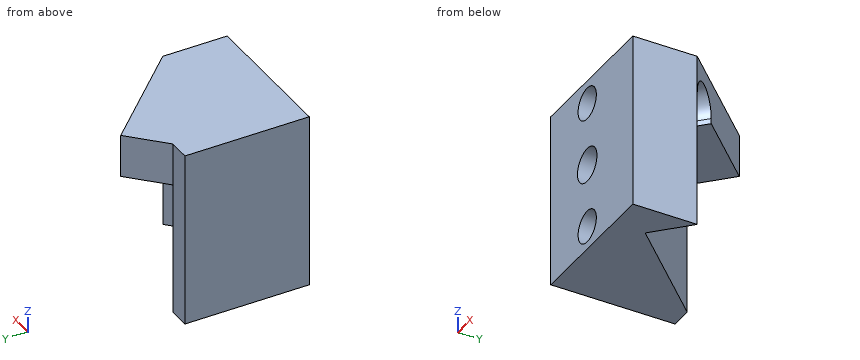
```python
from build123d import *

# Parameters (mm, degrees)
BOSS_EXTRUDE1_DEPTH       = 8.2
CUT_EXTRUDE1_DEPTH        = 2.2
SKETCH7_W                 = 6.75
SKETCH7_H                 = 8.2
BOSS_EXTRUDE2_DEPTH       = 1
F_1_5MM_DOWEL_HOLE1_D     = 1.5
F_1_5MM_DOWEL_HOLE1_DEPTH = 1.5
F_1_5MM_DOWEL_HOLE1_TIP   = 0.450645464
M2X0_4_TAPPED_HOLE1_D     = 1.6
M2X0_4_TAPPED_HOLE1_DEPTH = 2.5
M2X0_4_TAPPED_HOLE1_TIP   = 0.480688495


with BuildPart() as part:
    # Sketch1 → Boss-Extrude1 (new body)
    with BuildSketch(Plane.XY):
        Polygon((0, 0), (0, 4.787274917), (1, 4.787274917), (2.582547561, 6.315523332), (6.75, 2), (6.75, 0), align=None)
    extrude(amount=BOSS_EXTRUDE1_DEPTH)

    # Sketch2 → Cut-Extrude1 (cut)
    with BuildSketch(Plane(origin=(4.492176628, 4.338044544, 0), x_dir=(0, 0, -1), z_dir=(0.7193398, 0.69465837, 0))):
        with BuildLine():
            Line((0, -3.2502644), (-6.45, -3.2502644))
            ThreePointArc((-6.45, -3.2502644), (-7.45, -2.2502644), (-6.45, -1.2502644))
            Line((-6.45, -1.2502644), (-6.2, -1.2502644))
            Line((-6.2, -1.2502644), (-6.2, 3.2497356))
            Line((-6.2, 3.2497356), (0, 3.2497356))
            Line((0, 3.2497356), (0, -3.2502644))
        make_face()
    extrude(amount=-CUT_EXTRUDE1_DEPTH, mode=Mode.SUBTRACT)

    # Sketch7 → Boss-Extrude2 (add)
    with BuildSketch(Plane.XZ):
        with Locations((3.375, 4.1)):
            Rectangle(SKETCH7_W, SKETCH7_H)
    extrude(amount=BOSS_EXTRUDE2_DEPTH)

    # Ø1.5mm Dowel Hole1
    with Locations(Plane(origin=(0, -1, 0), x_dir=(-1, 0, 0), z_dir=(0, -1, 0))):
        with Locations((-3, -7.1), (-3, -1.1)):
            Hole(F_1_5MM_DOWEL_HOLE1_D / 2, depth=F_1_5MM_DOWEL_HOLE1_DEPTH)
            with Locations((0, 0, -(F_1_5MM_DOWEL_HOLE1_DEPTH + F_1_5MM_DOWEL_HOLE1_TIP / 2))):  # 118° drill point
                Cone(0, F_1_5MM_DOWEL_HOLE1_D / 2, F_1_5MM_DOWEL_HOLE1_TIP, mode=Mode.SUBTRACT)

    # M2x0.4 Tapped Hole1
    with Locations(Plane(origin=(0, -1, 0), x_dir=(-1, 0, 0), z_dir=(0, -1, 0))):
        with Locations((-3, -4.1)):
            Hole(M2X0_4_TAPPED_HOLE1_D / 2, depth=M2X0_4_TAPPED_HOLE1_DEPTH)
            with Locations((0, 0, -(M2X0_4_TAPPED_HOLE1_DEPTH + M2X0_4_TAPPED_HOLE1_TIP / 2))):  # 118° drill point
                Cone(0, M2X0_4_TAPPED_HOLE1_D / 2, M2X0_4_TAPPED_HOLE1_TIP, mode=Mode.SUBTRACT)


solid = part.part
```
Can you work these out from the model? Positions are in its coordinate system, mm. Coordinates: 2 decimals unless noted, no trailing zeros. Write each loop counter-clockwise with the first axis right and the second up, starting at its lowest first coordinate (ties: lowest second). Pieces come first, ordered by that corner, then holes. Notation, with made-up numbers: M 47.5,40.5 L 76.5,40.5 A8 ccw 76.5,47.5 Z; hole C -38,54.5 d9. An arc over 180 degrees is marked long. Write item = value, one per line. Start each with the question number.
Q1. If we section it at A-A, the plane y = -0.5: Write out the boundary of the cut face in (x, z).
Q2. I'm going to push flat-ended pins straight in: pin 1 (2 mm diameter, centred on x = 4, y = 3, fed in from -Z); pin 2 (1.8 mm diameter, centred on x = 3, z = 4.1, fed in from +Y); pin 3 (0.9 mm diameter, centred on x = 3, z = 1.1, fed in from -Y); pin 4 (1.5 mm diameter, centred on x = 3, y = 4, fed in from -Z). Where does each tip first touch, or does it pass through?
Q3. If we section it at B-B, the plane z = 6: Write out the boundary of the cut face in (x, y).
Q4. If we section it at D-D, the plane y = 6: Write out the boundary of the cut face in (x, z), then the cut area to 3 significant figures.
Q5. If we section it at C-C, the plane x = 1.75: Write out the boundary of the cut face in (y, z).
Q6. If I drill on L1, parallel to Z at x = 3, y = 0.3; L2, parallel to X at y = 0.4, z = 4.1; L3, parallel to Y at x = 2, z = 4.75, over which ranges is the centre line in solid material (lowest first)? Write a range as [from, to].
Check sheet entries:
q1.outline = M 0,0 L 6.75,0 L 6.75,8.2 L 0,8.2 Z; hole C 3,4.1 d1.6; hole C 3,1.1 d1.5; hole C 3,7.1 d1.5
q2.pin_1 = 0
q2.pin_2 = 3.65
q2.pin_3 = 0.68
q2.pin_4 = 6.2
q3.outline = M 0,-1 L 6.75,-1 L 6.75,2 L 5.17,0.47 L 1,4.79 L 0,4.79 Z
q4.outline = M 2.26,6.2 L 2.89,6.2 L 2.89,8.2 L 2.26,8.2 Z
q4.area = 1.26 mm²
q5.outline = M -1,0 L 4.01,0 L 4.01,6.2 L 5.51,6.2 L 5.51,8.2 L -1,8.2 Z
q6.L1 = [0, 0.35], [1.85, 3.3], [4.9, 6.35], [7.85, 8.2]
q6.L2 = [0, 2.2], [3.8, 6.75]
q6.L3 = [-1, 3.75]
